Verification items for the finished model (mm, model axes). Give positions to 0.01 mm unless a question says otherwise; leave off trailing zeros. Loops run counter-clockwise (first coordinate to the right, second up) from the corner with the lowest first, then second, coordinate; pieces in that order, holes last. Notation, with made-up numbers: M -3,54.5 L 28,54.5 A17 cw 28,68.5 Z; hole C 5.5,86.5 d5. An arc over 180 degrees is marked long. Use a Markdown table: item, result.
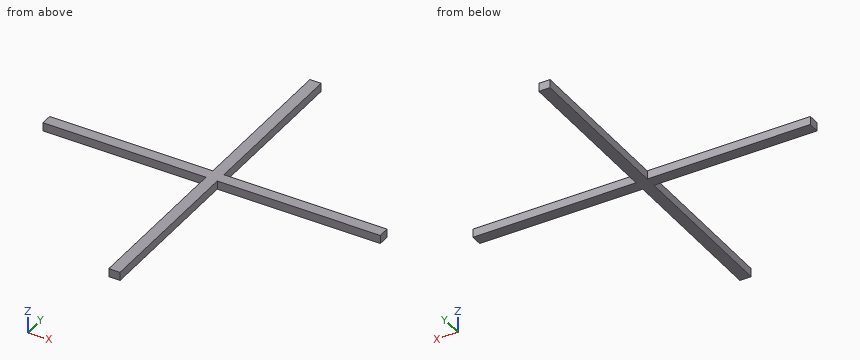
from build123d import *

# Parameters (mm, degrees)
F0_W     = 58
F0_H     = 4
F0_W_2   = 4
F0_H_2   = 58
F1_DEPTH = 3


with BuildPart() as f1:
    # F0 (on Top) → F1 (new body)
    with BuildSketch(Plane.XY):
        with Locations((-31, 0)):
            Rectangle(F0_W, F0_H)
        with Locations((0, -31)):
            Rectangle(F0_W_2, F0_H_2)
        Rectangle(F0_W_2, F0_H)
        with Locations((0, 31)):
            Rectangle(F0_W_2, F0_H_2)
        with Locations((31, 0)):
            Rectangle(F0_W, F0_H)
    extrude(amount=F1_DEPTH)


solid = f1.part
(1) Cross-section at B-B on x = 45.5. Record the cut outline in (y, z), then the cut area to 3 significant figures.
Results below:
| item | result |
|---|---|
| outline | M -2,0 L 2,0 L 2,3 L -2,3 Z |
| area | 12.0 mm^2 |
(2) Cross-section at A-A on z = 1.75. Record the cut outline in (x, y).
Results below:
| item | result |
|---|---|
| outline | M -60,-2 L -2,-2 L -2,-60 L 2,-60 L 2,-2 L 60,-2 L 60,2 L 2,2 L 2,60 L -2,60 L -2,2 L -60,2 Z |
(3) Gauge pin test, flat ends, axial feed: P1, Ø1.5, axis at y = -34.5, z = 1.5, coming from the -X side; P2, Ø0.9, axis at y = -24.5, z = 1.5, coming from the +X side; P3, Ø1.5, axis at x = 27.5, z = 2, coming from the +Y side; P4, Ø10, axis at x = 11.5, y = 36, coming from the -Z side. Record the tip position at first contact, or that the pin passes through.
Results below:
| item | result |
|---|---|
| P1 | x = -2 |
| P2 | x = 2 |
| P3 | y = 2 |
| P4 | through |
(4) Material ranges on line 1 (X direction, y = 13, z = 2.45), recorded low to high.
Results below:
| item | result |
|---|---|
| line 1 | -2 to 2 |
